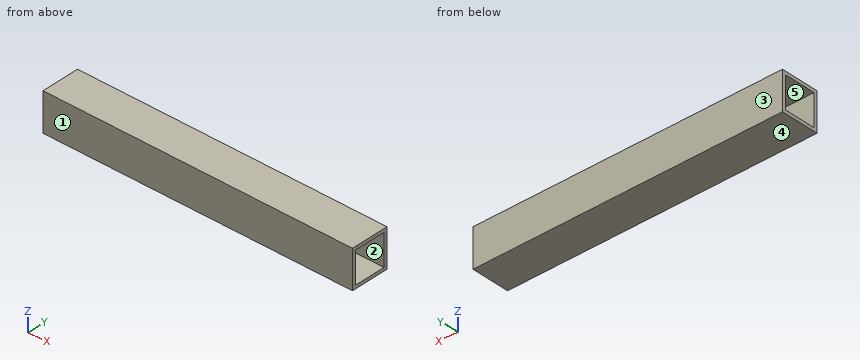
from build123d import *

# Parameters (mm, degrees)
SKETCH_W   = 31.75
SKETCH_H   = 31.75
SKETCH_W_2 = 26.2128
SKETCH_H_2 = 26.2128
PAD_DEPTH  = 257.175


with BuildPart() as part:
    # Sketch → Pad (new body)
    with BuildSketch(Plane.YZ):
        Rectangle(SKETCH_W, SKETCH_H)
        Rectangle(SKETCH_W_2, SKETCH_H_2, mode=Mode.SUBTRACT)
    extrude(amount=-PAD_DEPTH)


solid = part.part
Input: part model. Units: mm. Frame: model coordinates. Face numbers are marked on the shaded views. A direction names the side the tool comes from. Give positions to 0.01 mm unless a question says otherwise; leave off trailing zeros. Write each loop counter-clockwise with the first axis right and the second up, starting at its lowest first coordinate (ties: lowest second). Pieces come first, ordered by that corner, then holes.
Q1. First-contact query: P1, Ø10, axis at y = 3, z = 8.5, coming from the +X side; P2, Ø1, axis at y = 11.5, z = 4, coming from the +X side. Flat tips, straight axial feed; report the tip coordinate or a pass-through.
Q2. Pull-direction query (Z, two-part tool) for the marked faces 3, 4 and 5; classes: pulls with the +Z half, pulls with the -Z half, needs draft (parallel to the pull), parting line crosses it, or undercut.
Q3. Set-up query: the marked faces 1 and 2. Return all of +Z, -Z, +X, -X, +Y, -Y with unobstructed straight access to the full face (end or side cutting, diameter ignored); none if empty.
Q4. Section B-B, the plane z = -5.5. Output: boundary loops of the cut face in (x, y) (3 decimals), plus the area to 3 significant figures.
Q5. Section A-A, the plane x = -203.5. Output: boundary loops of the cut face in (y, z) (3 decimals).
Q6. Material intervals for probe 1 along Y at (x, z) = (-31.5, -5) (3 decimals), sorted ascending.
Filled in:
1. P1: stops at x = 0
1. P2: passes through
2. face 3: needs draft
2. face 4: pulls with the -Z half
2. face 5: undercut
3. face 1: +Z, -Z, +X, -X, -Y
3. face 2: +X, -X
4. outline: (-257.175, -15.875) - (0, -15.875) - (0, -13.106) - (-257.175, -13.106) - close; (-257.175, 13.106) - (0, 13.106) - (0, 15.875) - (-257.175, 15.875) - close
4. area: 1,420 mm2
5. outline: (-15.875, -15.875) - (15.875, -15.875) - (15.875, 15.875) - (-15.875, 15.875) - close; hole (-13.106, -13.106) - (13.106, -13.106) - (13.106, 13.106) - (-13.106, 13.106) - close
6. probe 1: y = -15.875 to -13.106, 13.106 to 15.875
